Part model, mm, in its own coordinate system. Round coordinates to 2 decimals unless told otherwise and drop trailing zeros. Loops run counter-clockwise (first coordinate to the right, second up) from the corner with the lowest first, then second, coordinate; pieces in that order, holes last. Notation, with made-up numbers: M -12,83.25 L 28,83.25 A31 cw 28,116.25 Z; hole C 45.25,88.5 d8. An arc over 180 degrees is marked long. Answer as CSV lines item,"result". Start each with the question number.
Item 1: Band-saw the part on C-C (x = 74). Give the cut face in (y, z), and give its area (3 significant figures).
Item 2: Band-saw the part on A-A (y = 165.1). Give the cut face in (x, z) (3 decimals), and give its area (3 significant figures).
Item 3: Drop flat-ended pins along their axis: pin 1 Ø20.5 at (x, y) = (21, 162) entering from -Z; pin 2 Ø20.5 at (x, y) = (18, 165.5) entering from +Z; pin 3 Ø3 at (y, z) = (128, -115) entering from +X (3 decimals). Give the stop position or say it passes through.
Item 4: Band-saw the part on B-B (z = -165.1). Give the cut face in (x, y) (3 decimals), and give its area (3 significant figures).
Item 5: Band-saw the part on D-D (x = 12). Give the cut face in (y, z), and give its area (3 significant figures).
Item 6: Wall check: line 1 (X direction, y = 194, z = -222.5) (3 decimals); line 2 (Z direction, x = 42.5, y = 140); line 3 (Y direction, x = 46.5, z = -164). Give the ranges that are in metal, low to high.
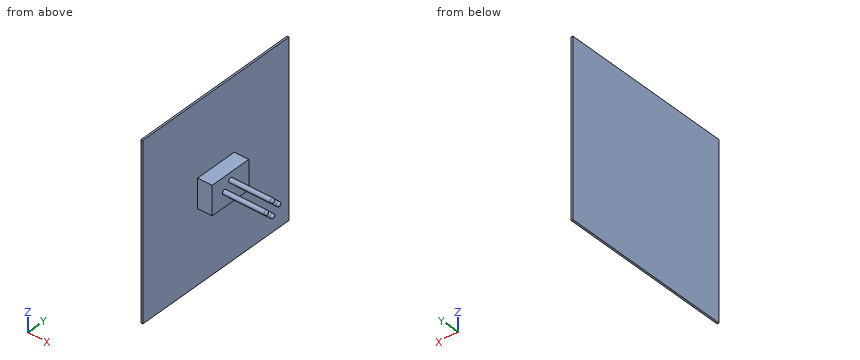
```python
from build123d import *

# Parameters (mm, degrees)
SKETCH1_W           = 304.8
SKETCH1_H           = 304.8
BOSS_EXTRUDE1_DEPTH = 3.175
SKETCH2_W           = 50.8
SKETCH2_H           = 76.2
BOSS_EXTRUDE2_DEPTH = 25.4
SKETCH3_R           = 3.937
BOSS_EXTRUDE3_DEPTH = 76.2
FILLET2_R           = 3.937


with BuildPart() as part:
    # Sketch1 → Boss-Extrude1 (new body)
    with BuildSketch(Plane(origin=(0, 0, 0), x_dir=(0, 0, -1), z_dir=(1, 0, 0))):
        with Locations((152.4, 152.4)):
            Rectangle(SKETCH1_W, SKETCH1_H)
    extrude(amount=BOSS_EXTRUDE1_DEPTH)

    # Sketch2 → Boss-Extrude2 (add)
    with BuildSketch(Plane(origin=(3.175, 0, 0), x_dir=(0, 0, -1), z_dir=(1, 0, 0))):
        with Locations((152.4, 152.4)):
            Rectangle(SKETCH2_W, SKETCH2_H)
    extrude(amount=BOSS_EXTRUDE2_DEPTH)

    # Sketch3 → Boss-Extrude3 (add)
    with BuildSketch(Plane(origin=(28.575, 0, 0), x_dir=(0, 0, -1), z_dir=(1, 0, 0))):
        with Locations(Location((152.4, 139.7, 0), (0, 0, 180))):
            Circle(SKETCH3_R)
        with Locations(Location((165.1, 152.4, 0), (0, 0, 180))):
            Circle(SKETCH3_R)
        with Locations(Location((152.4, 165.1, 0), (0, 0, 180))):
            Circle(SKETCH3_R)
        with Locations(Location((139.7, 152.4, 0), (0, 0, 180))):
            Circle(SKETCH3_R)
    extrude(amount=BOSS_EXTRUDE3_DEPTH)

    # Fillet2
    fillet2_edges = [part.edges().sort_by_distance(p)[0] for p in [
        (104.775, 139.7, -156.337),
        (104.775, 152.4, -169.037),
        (104.775, 165.1, -156.337),
        (104.775, 152.4, -143.637),
    ]]
    fillet(fillet2_edges, radius=FILLET2_R)


solid = part.part
```
Answer block:
1,outline,"C 139.7,-152.4 d7.87; C 152.4,-165.1 d7.87; C 152.4,-139.7 d7.87; C 165.1,-152.4 d7.87"
1,area,"195 mm^2"
2,outline,"M 0,-304.8 L 3.175,-304.8 L 3.175,-177.8 L 28.575,-177.8 L 28.575,-156.337 L 100.838,-156.337 A3.937 ccw 100.838,-148.463 L 28.575,-148.463 L 28.575,-127 L 3.175,-127 L 3.175,0 L 0,0 Z"
2,area,"2,850 mm^2"
3,pin 1,"stops at z = -177.8"
3,pin 2,"stops at z = -127"
3,pin 3,"stops at x = 3.175"
4,outline,"M 0,0 L 3.175,0 L 3.175,114.3 L 28.575,114.3 L 28.575,148.463 L 100.838,148.463 A3.937 ccw 100.838,156.337 L 28.575,156.337 L 28.575,190.5 L 3.175,190.5 L 3.175,304.8 L 0,304.8 Z"
4,area,"3,500 mm^2"
5,outline,"M 114.3,-177.8 L 190.5,-177.8 L 190.5,-127 L 114.3,-127 Z"
5,area,"3,870 mm^2"
6,line 1,"x = 0 to 3.175"
6,line 2,"z = -156.33 to -148.47"
6,line 3,"y = 148.62 to 156.18"
